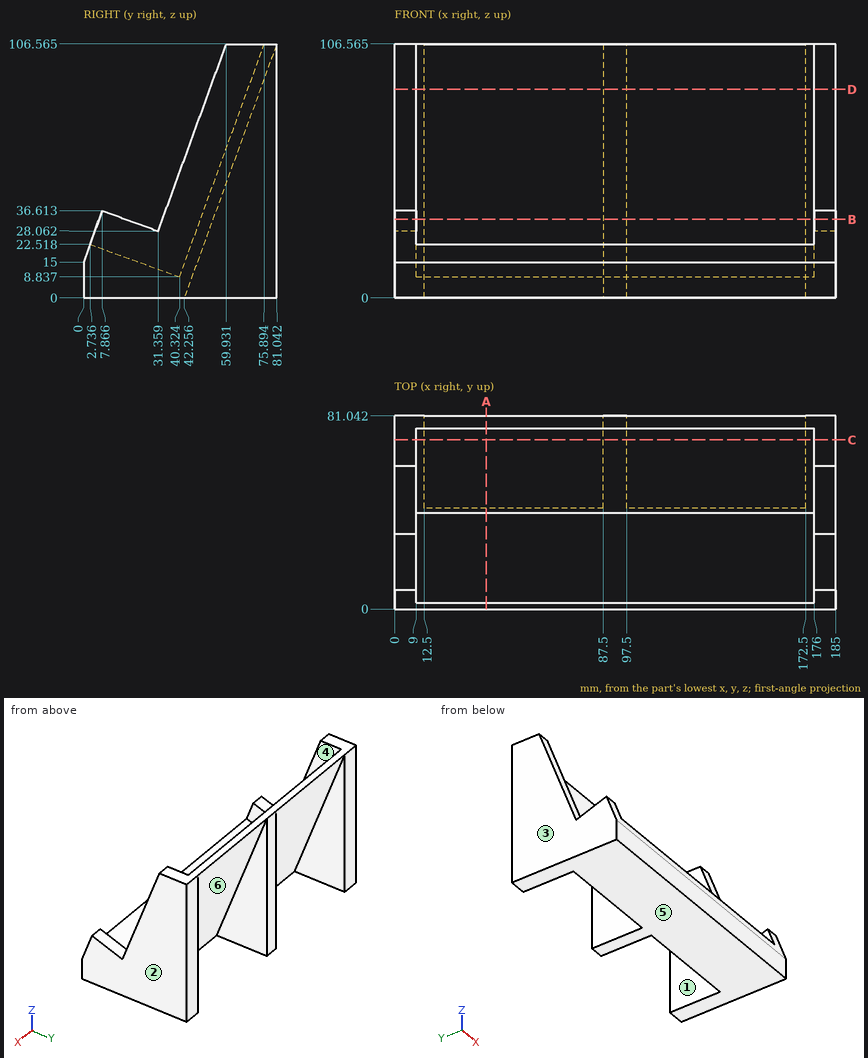
Input: dimensioned drawing with shaded views. Units: mm. Origin: part minimum x, y, z. A direction names the side the tool comes from. Round coordinates to 2 decimals unless told otherwise and drop trailing zeros. Order: outer loops, then holes, each group sorted by start corner. A loop starts at its lowest first (then second) coordinate and runs counter-clockwise, first axis right, second up. Notation, with made-up numbers: (32.25, 4.25) -> (42.25, 4.25) arc R26 cw to (42.25, 38.25) -> close; hole circle Ø9 at (-27, 68.25). An arc over 180 degrees is marked (long way). One line per item, written item: value. Start each with the question number.
Q1. Section query D-D (z = 87.5). Return the cut outline in (x, y) (1 decimal), plus the area to 3 significant figures.
Q2. Section query A-A (x = 38.5). Return the cut outline in (y, z) (1 decimal), plus the area to 4 significant figures.
Q3. Section query B-B (z = 33). Return the cut outline in (x, y) (1 decimal).
Q4. Pin query (flat end, axial travel): pin 1 (4 mm diameter, centred on x = 77.5, z = 16, fed in from +Y); pin 2 (4 mm diameter, centred on x = 114.5, z = 90.5, fed in from -Y); pin 3 (1 mm diameter, centred on x = 150.5, y = 18.5, fed in from +Z). Return the tip coordinate at first contact, or that it passes through.
Q5. Access query for the marked faces 4, 5 and 6. Directions: +Z, -Z, +X, -X, +Y, -Y. A direction counts if a zero-diameter tool reaches every point of the face in a straight line with its end or side. Return the directions, or none.
Q6. Section query C-C (y = 71). Return the cut outline in (x, z) (1 decimal).
Q7. Material intervals for probe 1 along X at (y, z) = (55, 5.5); probe 2 along X at (y, z) = (19, 23.5); probe 3 along Y at (x, z) = (155, 60) (1 decimal), sorted ascending.
Q8. Draft query along X for the marked faces 1, 2 and 3. Return one class per face: pulls with the +X half, pulls with the -X half, needs draft (parallel to the pull), parting line crosses it, or undercut.
Findings below:
1. outline: (0, 53) -> (9, 53) -> (9, 69) -> (176, 69) -> (176, 53) -> (185, 53) -> (185, 81) -> (172.5, 81) -> (172.5, 74.1) -> (97.5, 74.1) -> (97.5, 81) -> (87.5, 81) -> (87.5, 74.1) -> (12.5, 74.1) -> (12.5, 81) -> (0, 81) -> close
1. area: 1,480 mm²
2. outline: (0, 0) -> (42.3, 0) -> (81, 106.6) -> (75.9, 106.6) -> (40.3, 8.8) -> (2.7, 22.5) -> (0, 15) -> close
2. area: 1,175 mm²
3. outline: (0, 6.6) -> (9, 6.6) -> (9, 17.8) -> (0, 17.8) -> close; (0, 33.2) -> (9, 33.2) -> (9, 49.1) -> (176, 49.1) -> (176, 33.2) -> (185, 33.2) -> (185, 81) -> (172.5, 81) -> (172.5, 54.3) -> (97.5, 54.3) -> (97.5, 81) -> (87.5, 81) -> (87.5, 54.3) -> (12.5, 54.3) -> (12.5, 81) -> (0, 81) -> close; (176, 6.6) -> (185, 6.6) -> (185, 17.8) -> (176, 17.8) -> close
4. pin 1: y = 48.81
4. pin 2: y = 69.32
4. pin 3: z = 16.96
5. face 4: +Z
5. face 5: -Z, +X, -X, +Y, -Y
5. face 6: -Z, +Y
6. outline: (0, 0) -> (12.5, 0) -> (12.5, 79) -> (87.5, 79) -> (87.5, 0) -> (97.5, 0) -> (97.5, 79) -> (172.5, 79) -> (172.5, 0) -> (185, 0) -> (185, 106.6) -> (176, 106.6) -> (176, 93.1) -> (9, 93.1) -> (9, 106.6) -> (0, 106.6) -> close
7. probe 1: 0 to 12.5, 87.5 to 97.5, 172.5 to 185
7. probe 2: 0 to 9, 176 to 185
7. probe 3: 58.9 to 64.1
8. face 1: undercut
8. face 2: pulls with the +X half
8. face 3: pulls with the -X half
